Part model, mm, in its own coordinate system. Face numbers are marked on the shaded views. A direction names the side the tool comes from. Round coordinates to 2 decimals unless told otherwise and drop trailing zeros. Loops run counter-clockwise (first coordinate to the right, second up) from the corner with the lowest first, then second, coordinate; pieces in that order, holes last. Notation, with made-up numbers: (84.5, 62) -> (119.5, 62) arc R10 cw to (119.5, 78) -> close; hole circle Ø6 at (-27, -27.5). An arc over 180 degrees is marked (long way). Answer as CSV lines item,"result".
from build123d import *

# Parameters (mm, degrees)
SKETCH1_W            = 44.8
SKETCH1_H            = 2.99
BOSS_EXTRUDE1_DEPTH  = 44.8
FILLET1_RADIUS       = 1.495
FILLET1_LENGTH       = 44.8
M4_CLEARANCE_HOLE1_D = 4.8
M3_CLEARANCE_HOLE1_D = 3.4
SKETCH8_R            = 1.7
BOSS_EXTRUDE2_DEPTH  = 4
REVOLVE1_ANGLE       = 180
REVOLVE2_ANGLE       = 180


with BuildPart() as part:
    # Sketch1 → Boss-Extrude1 (new body)
    with BuildSketch(Plane(origin=(0, 0, 0), x_dir=(1, 0, 0), z_dir=(0, 1, 0))):
        Rectangle(SKETCH1_W, SKETCH1_H)
    extrude(amount=BOSS_EXTRUDE1_DEPTH)

    # Fillet1: full round fillet: the end face becomes a half cylinder, R = half its width
    fillet1_face = Plane((0, 0, 0), x_dir=(-1, 0, 0), z_dir=(0, -1, 0))  # on the end face: x along it, z out of the body
    fillet1_slab = fillet1_face.offset(-FILLET1_RADIUS / 2) * Box(FILLET1_LENGTH, 2 * FILLET1_RADIUS, FILLET1_RADIUS, mode=Mode.PRIVATE)  # the body's end, R deep
    fillet1_round = Plane((0, 1.495, 0), x_dir=(0, -1, 0), z_dir=(-1, 0, 0)) * Cylinder(FILLET1_RADIUS, FILLET1_LENGTH, mode=Mode.PRIVATE)  # its axis R under the face
    add(fillet1_slab - fillet1_round, mode=Mode.SUBTRACT)

    # M4 Clearance Hole1 (through all)
    with Locations(Plane.XY.offset(1.495)):
        with Locations((-17.5, 40.4), (-17.5, 20.4), (17.5, 20.4), (17.5, 40.4)):
            Hole(M4_CLEARANCE_HOLE1_D / 2)

    # M3 Clearance Hole1 (through all)
    with Locations(Plane.XY.offset(1.495)):
        with Locations((0, 8.2)):
            Hole(M3_CLEARANCE_HOLE1_D / 2)

    # Sketch8 → Boss-Extrude2 (add)
    with BuildSketch(Plane.XY.offset(1.495)):
        with Locations(Location((-7.5, 8.2, 0), (0, 0, 180))):
            Circle(SKETCH8_R)
        with Locations(Location((7.5, 8.2, 0), (0, 0, 180))):
            Circle(SKETCH8_R)
    extrude(amount=BOSS_EXTRUDE2_DEPTH)

    # Sketch9 → Revolve1 (revolve)
    with BuildSketch(Plane.XY.offset(5.495)):
        with BuildLine():
            Line((-7.5, 9.9), (-7.5, 6.5))
            ThreePointArc((-7.5, 6.5), (-5.8, 8.2), (-7.5, 9.9))
        make_face()
    revolve(axis=Axis((-7.5, 9.9, 5.495), (0, -1, 0)), revolution_arc=REVOLVE1_ANGLE)

    # Sketch10 → Revolve2 (revolve)
    with BuildSketch(Plane.XY.offset(5.495)):
        with BuildLine():
            Line((7.5, 9.9), (7.5, 6.5))
            ThreePointArc((7.5, 6.5), (9.2, 8.2), (7.5, 9.9))
        make_face()
    revolve(axis=Axis((7.5, 9.9, 5.495), (0, -1, 0)), revolution_arc=REVOLVE2_ANGLE)


solid = part.part
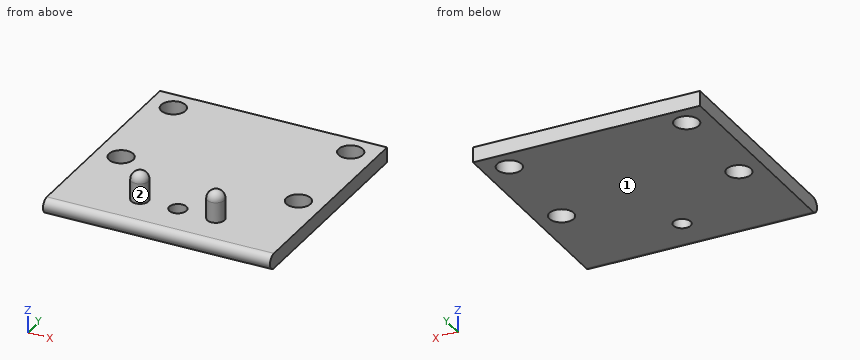
Q1. Drop a flat-ended pin along its axis: P1, Ø4, axis at x = 0, y = 8.2, coming from the +Z side (3 decimals). Give the stop position or say it passes through.
Geometry results:
P1,"z = 1.495"
Q2. Saw through at A-A, the plane x = -17.5. Write the cut outline in (y, z) (3 decimals), then the cut area to 3 significant figures.
Geometry results:
outline,"(1.495, -1.495) -> (18, -1.495) -> (18, 1.495) -> (1.495, 1.495) arc R1.495 ccw to start; (22.8, -1.495) -> (38, -1.495) -> (38, 1.495) -> (22.8, 1.495) -> close; (42.8, -1.495) -> (44.8, -1.495) -> (44.8, 1.495) -> (42.8, 1.495) -> close"
area,"104 mm2"
Q3. Drill centre lines: line 1 along Y through (x, z) = (-17.5, -0.3); line 2 along Y through (x, z) = (-17.5, 0.6); line 3 along Z through (x, y) = (-1, 18) (3 decimals). Where is each one in solid material? Low to high.
Geometry results:
line 1,"0.03 to 18, 22.8 to 38, 42.8 to 44.8"
line 2,"0.13 to 18, 22.8 to 38, 42.8 to 44.8"
line 3,"-1.495 to 1.495"
Q4. Saw through at C-C, the plane z = 0. Write the cut outline in (x, y).
Geometry results:
outline,"(-22.4, 0) -> (22.4, 0) -> (22.4, 44.8) -> (-22.4, 44.8) -> close; hole circle Ø4.8 at (-17.5, 20.4); hole circle Ø4.8 at (-17.5, 40.4); hole circle Ø3.4 at (0, 8.2); hole circle Ø4.8 at (17.5, 20.4); hole circle Ø4.8 at (17.5, 40.4)"
Q5. Saw through at B-B, the plane y = 20.4. Write the cut outline in (x, z) (3 decimals), then the cut area to 3 significant figures.
Geometry results:
outline,"(-22.4, -1.495) -> (-19.9, -1.495) -> (-19.9, 1.495) -> (-22.4, 1.495) -> close; (-15.1, -1.495) -> (15.1, -1.495) -> (15.1, 1.495) -> (-15.1, 1.495) -> close; (19.9, -1.495) -> (22.4, -1.495) -> (22.4, 1.495) -> (19.9, 1.495) -> close"
area,"105 mm2"
Q6. Which spindle directions (+Z, -Z, +X, -X, +Y, -Y) get a long thin tool onto all of the face, cutting with end or side? Do the marked faces 1 and 2. Say none if no direction does.
Geometry results:
face 1,"-Z, +X, -X, +Y, -Y"
face 2,"+Z"
Q7. Saw through at D-D, the plane z = 3.25. Write the cut outline in (x, y).
Geometry results:
outline,"circle Ø3.4 at (-7.5, 8.2); circle Ø3.4 at (7.5, 8.2)"
